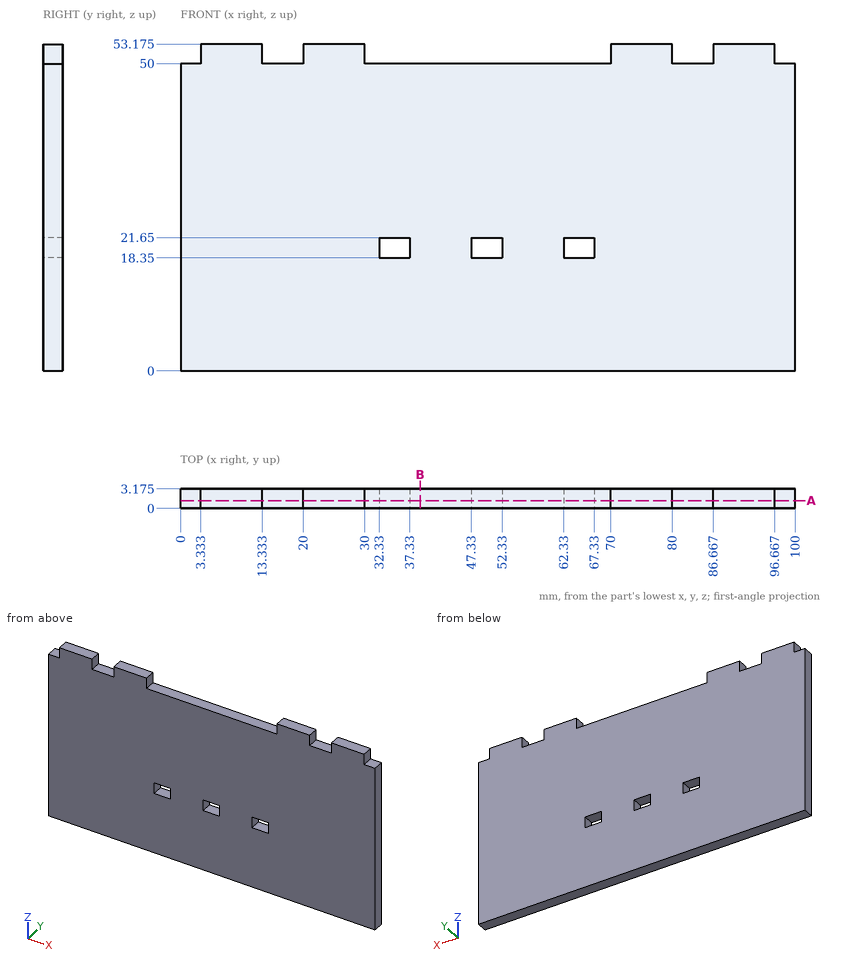
Check sheet for the drawn part. Datum: minimum x, y, z corner. Units: mm. Round coordinates to 2 decimals unless told otherwise and drop trailing zeros. Order: outer loops, then holes, each group sorted by start corner. A loop starts at its lowest first (then second) coordinate and runs counter-clockwise, first axis right, second up. Notation, with made-up numbers: (38, 24.25) -> (51, 24.25) arc R30 ccw to (51, 52.25) -> close; hole circle Ø6 at (-1, -36). An arc over 180 degrees is marked (long way). Return JSON: item names as keys, results as strings. Group by question number.
Q1. Gauge pin test, flat ends, axial feed: pin 1 (1.6 mm diameter, centred on y = 2, z = 51, fed in from -X); pin 2 (1.6 mm diameter, centred on x = 2.5, y = 2, fed in from +Z); pin 3 (1 mm diameter, centred on y = 1, z = 51, fed in from +X). Record the tip position at first contact, or that the pin passes through.
Q2. Section check B-B, the plane x = 39. Record the boundary of the cut face in (y, z) (1 decimal), plus the area to 3 significant figures.
Q3. Material ranges on probe 1 along X at (y, z) = (1.45, 21.5); probe 2 along Z at (x, y) = (49, 2.4); probe 3 along Z at (x, y) = (16.5, 0.9), recorded low to high. Write a range as from..to.
Q4. Section check A-A, the plane y = 1.25. Count the separate pieces of the cut face and the enclosed holes in it, plus the area to 3 significant figures.
Numbers:
{
 "1": {"pin 1": "x = 3.33", "pin 2": "z = 50", "pin 3": "x = 96.67"},
 "2": {"outline": "(0, 0) -> (3.2, 0) -> (3.2, 50) -> (0, 50) -> close", "area": "159 mm^2"},
 "3": {"probe 1": "0..32.33, 37.33..47.33, 52.33..62.33, 67.33..100", "probe 2": "0..18.35, 21.65..50", "probe 3": "0..50"},
 "4": {"separate pieces": "1", "enclosed holes": "3", "area": "5,080 mm^2"}
}
